For this review, use the dimensioned drawing (mm, ordinates from the lowest corner) and the shaded views. A direction names the side the tool comes from. Round coordinates to 2 decimals unless told otherwise and drop trailing zeros. Order: outer loops, then holes, each group sorted by start corner. A loop starts at its lowest first (then second) coordinate and runs counter-clockwise, first axis right, second up. Notation, with made-up numbers: (-5, -40) -> (33, -40) arc R24 ccw to (33, -6) -> close; hole circle Ø9 at (-28.75, 28). An arc over 180 degrees is marked (long way). Answer in a Markdown table with one row per item.
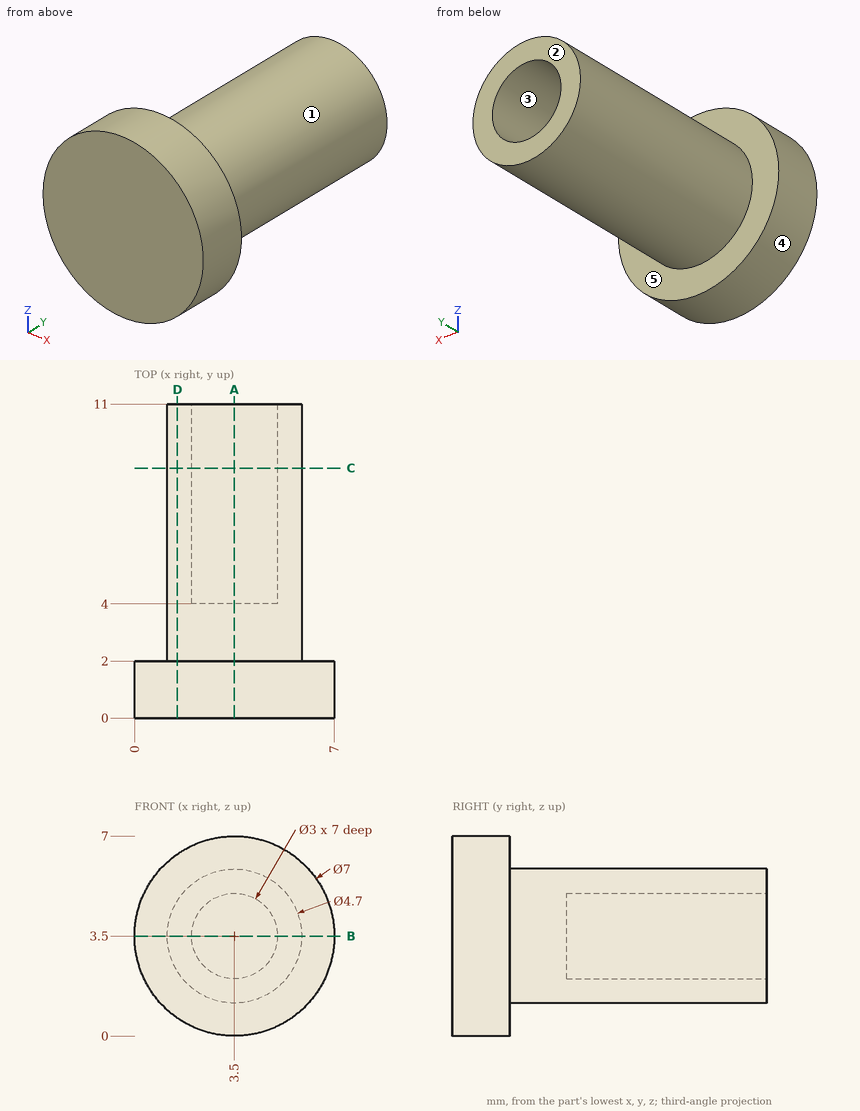
Q1. The part is to be moulded in two halves that separate along X. For the marked faces 1, 2 and 3, say which applies: +X half, -X half, draft (parallel to the pull), parting line (faces both ways), or undercut.
Answer key:
| item | result |
|---|---|
| face 1 | parting line |
| face 2 | draft |
| face 3 | undercut |
Q2. Take a section at C-C, the plane y = 8.75. Write out the cut boundary in (x, z), then the cut area to 3 significant figures.
Answer key:
| item | result |
|---|---|
| outline | circle Ø4.7 at (3.5, 3.5); hole circle Ø3 at (3.5, 3.5) |
| area | 10.3 mm^2 |
Q3. Tool access review of the marked faces 4 and 5: name each direction out of +Z, -Z, +X, -X, +Y, -Y from which nothing blocks a thin tool from reaching the whole face with its end or side.
Answer key:
| item | result |
|---|---|
| face 4 | +Y, -Y |
| face 5 | +Y |
Q4. Take a section at A-A, the plane x = 3.5. Write out the cut boundary in (y, z).
Answer key:
| item | result |
|---|---|
| outline | (0, 0) -> (2, 0) -> (2, 1.15) -> (11, 1.15) -> (11, 2) -> (4, 2) -> (4, 5) -> (11, 5) -> (11, 5.85) -> (2, 5.85) -> (2, 7) -> (0, 7) -> close |
Q5. Take a section at D-D, the plane x = 1.5. Write out the cut boundary in (y, z), then the cut area to 3 significant figures.
Answer key:
| item | result |
|---|---|
| outline | (0, 0.63) -> (2, 0.63) -> (2, 2.27) -> (11, 2.27) -> (11, 4.73) -> (2, 4.73) -> (2, 6.37) -> (0, 6.37) -> close |
| area | 33.7 mm^2 |
Q6. To check wall thickness, follow probe 1 along Z at (x, y) = (3.5, 8); probe 2 along Y at (x, z) = (2.75, 0.5); probe 3 along Z at (x, y) = (4, 9.75). State the ranges of each line that lie inside material, in increasing order.
Answer key:
| item | result |
|---|---|
| probe 1 | z = 1.15 to 2, 5 to 5.85 |
| probe 2 | y = 0 to 2 |
| probe 3 | z = 1.2 to 2.09, 4.91 to 5.8 |
Q7. Take a section at B-B, the plane z = 3.5. Write out the cut boundary in (x, y).
Answer key:
| item | result |
|---|---|
| outline | (0, 0) -> (7, 0) -> (7, 2) -> (5.85, 2) -> (5.85, 11) -> (5, 11) -> (5, 4) -> (2, 4) -> (2, 11) -> (1.15, 11) -> (1.15, 2) -> (0, 2) -> close |
